Here's how the part is built. I have some questions about the finished solid (model axes, mm). A direction names the side the tool comes from. Round coordinates to 2 decimals unless told otherwise and drop trailing zeros. Loops run counter-clockwise (first coordinate to the right, second up) from the corner with the lowest first, then second, coordinate; pieces in that order, holes last. Notation, with made-up numbers: (-17.75, 21.5) - (-9.75, 21.5) arc R31 cw to (-9.75, 46.5) - close; hole circle Ø10 at (-4.5, 20). An arc over 180 degrees is marked (long way). Answer as a JSON object with one key per item and string values. Group by question number.
1) I want a section at B-B, the plane y = 106.5. Please give me the cut outline in (x, z), then the cut area to 3 significant figures.
2) Which directions (+Z, -Z, +X, -X, +Y, -Y) give clear straight access to the entire face, cutting with the end or side of a thin tool? Please do faces 1 (the face through (-138, 74, 2)), 2 (the face through (-125, 146, 9)), 3 (the face through (140, 74.6, 135.2)).
3) Will these pins go through, and if not, where does the flat tip stop? P1, Ø12, axis at y = 28.5, z = 28, coming from the +X side; P2, Ø4.5, axis at x = -51.5, y = 2, coming from the -Z side; P3, Ø5.5, axis at y = 2, z = -36.5, coming from the +X side; P4, Ø2, axis at x = 16.5, y = 1.5, coming from the +Z side.
4) I want a section at C-C, the plane z = 51. Please give me the cut outline in (x, y).
5) I want a section at A-A, the plane x = 96.5. Please give me the cut outline in (y, z).
6) If we mould it in two halves opening along Y, with no side actions, what happens to faces 4 (the face through (-130, 5, 20)), 5 (the face through (-3, 76, -140)), 6 (the face through (-130, 141, 20)), 7 (the face through (-125, 0, 9))? For each: pulls with the +Y half, pulls with the -Y half, needs draft (parallel to the pull), parting line crosses it, or undercut.
7) If I drill on line 1 along Z through (x, y) = (104, 88); line 2 along Y through (x, z) = (-110, 121.5); line 3 along X through (y, z) = (79.5, -39), over which ranges is the centre line in solid material (lowest first)? Write a range as [from, to].
from build123d import *

# Parameters (mm, degrees)
SKETCH_1_W          = 280
SKETCH_1_H          = 280
EXTRUDE_1_DEPTH     = 150
SKETCH_2_W          = 280
SKETCH_2_H          = 272
CUT_EXTRUDE_1_DEPTH = 4
SKETCH_3_W          = 280
SKETCH_3_H          = 4
CUT_EXTRUDE_2_DEPTH = 4
SKETCH_4_W          = 270
SKETCH_4_H          = 136
CUT_EXTRUDE_3_DEPTH = 278
SKETCH_6_W          = 260
SKETCH_6_H          = 232
CUT_EXTRUDE_7_DEPTH = 247
FILLET_4_R          = 2
FILLET_5_R          = 2
FILLET_6_R          = 2
FILLET_7_R          = 2


with BuildPart() as part:
    # 草图1 → 凸台-拉伸1 (new body)
    with BuildSketch(Plane(origin=(0, 0, 0), x_dir=(1, 0, 0), z_dir=(0, 1, 0))):
        Rectangle(SKETCH_1_W, SKETCH_1_H)
    extrude(amount=EXTRUDE_1_DEPTH)

    # 草图2 → 切除-拉伸1 (cut)
    with BuildSketch(Plane(origin=(0, 150, 0), x_dir=(1, 0, 0), z_dir=(0, 1, 0))):
        Rectangle(SKETCH_2_W, SKETCH_2_H)
    extrude(amount=-CUT_EXTRUDE_1_DEPTH, mode=Mode.SUBTRACT)

    # 草图3 → 切除-拉伸2 (cut)
    with BuildSketch(Plane.XZ):
        with Locations((0, 138)):
            Rectangle(SKETCH_3_W, SKETCH_3_H)
        with Locations((0, -138)):
            Rectangle(SKETCH_3_W, SKETCH_3_H)
    extrude(amount=-CUT_EXTRUDE_2_DEPTH, mode=Mode.SUBTRACT)

    # 草图4 → 切除-拉伸3 (cut)
    with BuildSketch(Plane(origin=(140, 0, 0), x_dir=(0, 0, -1), z_dir=(1, 0, 0))):
        with Locations((0, 73)):
            Rectangle(SKETCH_4_W, SKETCH_4_H)
    extrude(amount=-CUT_EXTRUDE_3_DEPTH, mode=Mode.SUBTRACT)

    # 草图6 → 切除-拉伸7 (cut, through all)
    with BuildSketch(Plane(origin=(0, 146, 0), x_dir=(1, 0, 0), z_dir=(0, 1, 0))):
        with Locations((10, 0)):
            Rectangle(SKETCH_6_W, SKETCH_6_H)
    extrude(amount=-CUT_EXTRUDE_7_DEPTH, mode=Mode.SUBTRACT)

    # 圆角4
    fillet_4_edges = [part.edges().sort_by_distance(p)[0] for p in [
        (140, 77, -140),
        (140, 77, 140),
    ]]
    fillet(fillet_4_edges, radius=FILLET_4_R)

    # 圆角5
    fillet_5_edges = [part.edges().sort_by_distance(p)[0] for p in [
        (140, 146, 126),
        (140, 146, -126),
    ]]
    fillet(fillet_5_edges, radius=FILLET_5_R)

    # 圆角6
    fillet_6_edges = [part.edges().sort_by_distance(p)[0] for p in [
        (-120, 143.5, 116),
        (-120, 2.5, 116),
        (-120, 143.5, -116),
        (-120, 2.5, -116),
    ]]
    fillet(fillet_6_edges, radius=FILLET_6_R)

    # 圆角7
    fillet_7_edges = [part.edges().sort_by_distance(p)[0] for p in [
        (1, 5, 135),
        (1, 141, 135),
        (1, 141, -135),
        (1, 5, -135),
        (-138, 73, 135),
        (-138, 141, 0),
        (-138, 73, -135),
        (-138, 5, 0),
    ]]
    fillet(fillet_7_edges, radius=FILLET_7_R)


solid = part.part
Outcome:
{
 "1": {"outline": "(-140, -140) - (138, -140) arc R2 ccw to (140, -138) - (140, -135) - (-136, -135) arc R2 cw to (-138, -133) - (-138, 133) arc R2 cw to (-136, 135) - (140, 135) - (140, 138) arc R2 ccw to (138, 140) - (-140, 140) - close", "area": "3,340 mm^2"},
 "2": {"face 1": "+X", "face 2": "+X, -X, +Y", "face 3": "+Z, -Z, +X, +Y, -Y"},
 "3": {"P1": "x = -138", "P2": "z = -140", "P3": "x = -120", "P4": "z = 136"},
 "4": {"outline": "(-140, 0) - (-120, 0) - (-120, 5) - (-136, 5) arc R2 cw to (-138, 7) - (-138, 139) arc R2 cw to (-136, 141) - (-120, 141) - (-120, 146) - (-140, 146) - close"},
 "5": {"outline": "(0, -136) - (4, -136) - (4, -140) - (150, -140) - (150, -136) - (146, -136) - (146, -116) - (141, -116) - (141, -133) arc R2 cw to (139, -135) - (7, -135) arc R2 cw to (5, -133) - (5, -116) - (0, -116) - close; (0, 116) - (5, 116) - (5, 133) arc R2 cw to (7, 135) - (139, 135) arc R2 cw to (141, 133) - (141, 116) - (146, 116) - (146, 136) - (150, 136) - (150, 140) - (4, 140) - (4, 136) - (0, 136) - close"},
 "6": {"face 4": "undercut", "face 5": "needs draft", "face 6": "undercut", "face 7": "pulls with the -Y half"},
 "7": {"line 1": "[-140, -135], [135, 140]", "line 2": "[0, 5], [141, 146]", "line 3": "[-140, -138]"}
}
